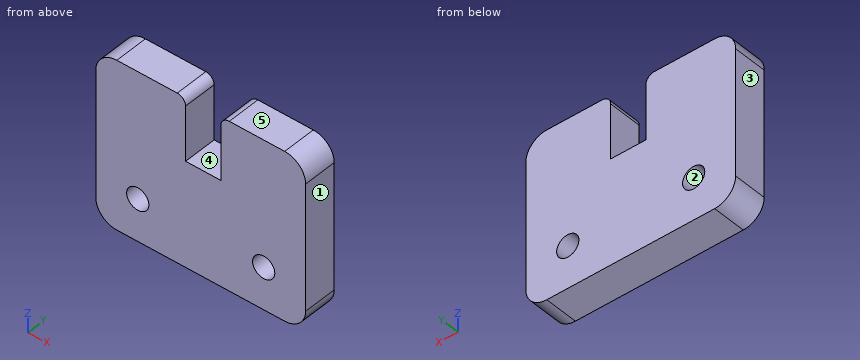
Autodesk Inventor part; units mm, degrees
ref_plane "YZ Plane" through (0, 0, 0) normal (1, 0, 0) x (0, 1, 0)
ref_plane "XZ Plane" through (0, 0, 0) normal (0, 1, 0) x (-1, 0, 0)
ref_plane "XY Plane" through (0, 0, 0) normal (0, 0, 1) x (1, 0, 0)
sketch "Sketch1" plane through (0, 0, 0) normal (0, 1, 0) x (-1, 0, 0)
  line L0 (0, 0) -> (20.2, 0)
  line L1 (50, 0) -> (50, -40)
  line L2 (50, -40) -> (0, -40)
  line L3 (0, -40) -> (0, 0)
  line L4 (20.2, 0) -> (20.2, -15)
  line L5 (20.2, -15) -> (28.6, -15)
  line L6 (28.6, -15) -> (28.6, 0)
  circle A0 centre (40, -30) radius 2.65
  circle A1 centre (10, -30) radius 2.65
  line L7 (28.6, 0) -> (50, 0)
  dimension "d0" = 40
  dimension "d1" = 50
  dimension "d2" = 8.4
  dimension "d3" = 15
  dimension "d4" = 20.2
  dimension "d5" = 5.3
  dimension "d6" = 5.3
  dimension "d7" = 10
  dimension "d8" = 10
  dimension "d9" = 10
  dimension "d10" = 10
extrude "Extrusion1" add sketch "Sketch1" along normal blind 8
fillet "Fillet1" radius 5 4 edges at (0, 4, -40) (-50, 4, -40) (0, 4, 0) (-50, 4, 0)
fillet "Fillet2" radius 2 2 edges at (-28.6, 4, 0) (-20.2, 4, 0)
Here's how the part is built. I have some questions about the finished solid (model axes, mm). Face numbers are marked on the shaded views. A direction names the side the tool comes from. Coordinates: 2 decimals unless noted, no trailing zeros. Write each loop counter-clockwise with the first axis right and the second up, starting at its lowest first coordinate (ties: lowest second). Pieces come first, ordered by that corner, then holes. Notation, with made-up numbers: (48.25, 2) -> (94.25, 2) arc R26 ccw to (94.25, 16) -> close; hole circle Ø5 at (18, -18.75). An arc over 180 degrees is marked (long way). Use a Markdown table: item, result. Add a question column.
(1) If we section it at C-C, the plane y = 3.5: Write out the boundary of the cut face in (x, z).
(2) If we section it at A-A, the plane z = -30: Write out the boundary of the cut face in (x, y).
(3) We'd pull the mould along X, two halves only. Please class the marked faces 1, 2 and 3: +X half, -X half, draft (parallel to the pull), parting line (faces both ways), or undercut.
(4) Please list where these lines run through material, in increasing order: line 1 (Z direction, x = -40, y = 5.5); line 2 (X direction, y = 5.5, z = -13.5); line 3 (X direction, y = 6.5, z = -32).
(5) For the marked faces 4 and 5, which set-ups out of +Z, -Z, +X, -X, +Y, -Y let a thin tool reach every point of the face, with its end or its side?
(6) If we section it at B-B, the plane x = -10: Write out the boundary of the cut face in (y, z).
(7) I'm going to push flat-ended pins straight in: P1, Ø2.5, axis at x = -26.5, y = 4, coming from the +Z side; P2, Ø2, axis at y = 2.5, z = -27.5, coming from the +X side. Where does each tip first touch, or does it pass through?
Outcome:
| question | item | result |
|---|---|---|
| 1 | outline | (-50, -35) arc R5 ccw to (-45, -40) -> (-5, -40) arc R5 ccw to (0, -35) -> (0, -5) arc R5 ccw to (-5, 0) -> (-18.2, 0) arc R2 ccw to (-20.2, -2) -> (-20.2, -15) -> (-28.6, -15) -> (-28.6, -2) arc R2 ccw to (-30.6, 0) -> (-45, 0) arc R5 ccw to (-50, -5) -> close; hole circle Ø5.3 at (-40, -30); hole circle Ø5.3 at (-10, -30) |
| 2 | outline | (-50, 0) -> (-42.65, 0) -> (-42.65, 8) -> (-50, 8) -> close; (-37.35, 0) -> (-12.65, 0) -> (-12.65, 8) -> (-37.35, 8) -> close; (-7.35, 0) -> (0, 0) -> (0, 8) -> (-7.35, 8) -> close |
| 3 | face 1 | +X half |
| 3 | face 2 | undercut |
| 3 | face 3 | -X half |
| 4 | line 1 | z = -40 to -32.65, -27.35 to 0 |
| 4 | line 2 | x = -50 to -28.6, -20.2 to 0 |
| 4 | line 3 | x = -50 to -41.74, -38.26 to -11.74, -8.26 to 0 |
| 5 | face 4 | +Z, +Y, -Y |
| 5 | face 5 | +Z, +X, -X, +Y, -Y |
| 6 | outline | (0, -40) -> (8, -40) -> (8, -32.65) -> (0, -32.65) -> close; (0, -27.35) -> (8, -27.35) -> (8, 0) -> (0, 0) -> close |
| 7 | P1 | stops at z = -15 |
| 7 | P2 | stops at x = 0 |
